```python
from build123d import *

# Parameters (mm, degrees)
F0_W     = 2000
F0_H     = 1000
F1_DEPTH = 25
F2_W     = 100
F2_H     = 100
F3_DEPTH = 700
F5_D     = 50
F5_DEPTH = 500.001
F6_D     = 50


with BuildPart() as f1:
    # F0 (on Top) → F1 (new body)
    with BuildSketch(Plane.XY):
        Rectangle(F0_W, F0_H)
    extrude(amount=F1_DEPTH)

    # F2 (on Top) → F3 (join)
    with BuildSketch(Plane.XY):
        with Locations((-900, 400)):
            Rectangle(F2_W, F2_H)
        with Locations((-900, -400)):
            Rectangle(F2_W, F2_H)
        with Locations((900, 400)):
            Rectangle(F2_W, F2_H)
        with Locations((900, -400)):
            Rectangle(F2_W, F2_H)
    extrude(amount=F3_DEPTH)

    # F5 (through all, one way)
    with BuildSketch(Plane(origin=(0, 0, 0), x_dir=(1, 0, 0), z_dir=(0, 1, 0))):
        with Locations((-900, -500), (-900, -300), (-900, -100)):
            Circle(F5_D / 2)
    extrude(amount=-F5_DEPTH, mode=Mode.SUBTRACT)

    # F6 (through all)
    with Locations(Plane.XZ):
        with Locations((-900, 300), (-900, 500), (-900, 100)):
            Hole(F6_D / 2)


solid = f1.part
```
Geometry check sheet. Reference: the model listing, model coordinates, mm. A direction names the side the tool comes from. Give positions to 0.01 mm unless a question says otherwise; leave off trailing zeros. Order: outer loops, then holes, each group sorted by start corner. A loop starts at its lowest first (then second) coordinate and runs counter-clockwise, first axis right, second up. Notation, with made-up numbers: (73, 84) - (129, 84) arc R26 ccw to (129, 107) - close; hole circle Ø1 at (57.5, -36.75). An arc over 180 degrees is marked (long way). Answer in a Markdown table with one row per item. Add a question column.
Q1. Cross-section at B-B, the plane z = 184.5. Enter the section's corners in (x, y), then the cut area to 3 significant figures.
Q2. Cross-section at C-C, the plane x = -900. Count the separate pieces of the cut face and the enclosed holes in it, then the cut area to 3 significant figures.
Q3. Gauge pin test, flat end, axial feed: pin 1 (8 mm diameter, centred on x = -110, y = 395, fed in from +Z). Record the tip position at first contact, or that the pin passes through.
Q4. Tool access check on faces 5 (the flat face through (-901, -450, 358)), 6 (the flat face through (-850, -401, 358)), 7 (the flat face through (-950, -401, 358)). Record the directions out of +Z, -Z, +X, -X, +Y, -Y that give a thin tool (end or side, any length) a straight path to the whole face; none if there is none.
Q5. Mould release check, pull along Y, two halves, no side actions. Record for faces 1 (the flat face through (850, 399, 358)), 2 (the flat face through (-901, 450, 358)), 3 (the flat face through (-901, 350, 358)), 4 (the flat face through (899, -350, 358)): pulls with the +Y half, pulls with the -Y half, needs draft (parallel to the pull), parting line crosses it, or undercut.
Q6. Cross-section at D-D, the plane y = -301. Enter the section's corners in (x, z).
Q7. Material ranges on probe 1 along Z at (x, y) = (-900, 414); probe 2 along X at (y, z) = (-402, 300); probe 3 along Y at (x, z) = (874, 594.5), recorded low to high. Write a range as from..to.
Q8. Cross-section at A-A, the plane z = 300. Enter the section's corners in (x, y), then the cut area to 3 significant figures.
Check values:
| question | item | result |
|---|---|---|
| 1 | outline | (-950, -450) - (-850, -450) - (-850, -350) - (-950, -350) - close; (-950, 350) - (-850, 350) - (-850, 450) - (-950, 450) - close; (850, -450) - (950, -450) - (950, -350) - (850, -350) - close; (850, 350) - (950, 350) - (950, 450) - (850, 450) - close |
| 1 | area | 40,000 mm^2 |
| 2 | separate pieces | 7 |
| 2 | enclosed holes | 0 |
| 2 | area | 130,000 mm^2 |
| 3 | pin 1 | stops at z = 25 |
| 4 | face 5 | +Z, +X, -X, -Y |
| 4 | face 6 | +Z, +Y, -Y |
| 4 | face 7 | +Z, -X, +Y, -Y |
| 5 | face 1 | needs draft |
| 5 | face 2 | pulls with the +Y half |
| 5 | face 3 | undercut |
| 5 | face 4 | undercut |
| 6 | outline | (-1000, 0) - (1000, 0) - (1000, 25) - (-1000, 25) - close |
| 7 | probe 1 | z = 0..75, 125..275, 325..475, 525..700 |
| 7 | probe 2 | x = -950..-925, -875..-850, 850..950 |
| 7 | probe 3 | y = -450..-350, 350..450 |
| 8 | outline | (-950, -450) - (-925, -450) - (-925, -350) - (-950, -350) - close; (-950, 350) - (-925, 350) - (-925, 450) - (-950, 450) - close; (-875, -450) - (-850, -450) - (-850, -350) - (-875, -350) - close; (-875, 350) - (-850, 350) - (-850, 450) - (-875, 450) - close; (850, -450) - (950, -450) - (950, -350) - (850, -350) - close; (850, 350) - (950, 350) - (950, 450) - (850, 450) - close |
| 8 | area | 30,000 mm^2 |
